The model under review builds one solid part; all positions refer to its coordinate system, in mm. A direction names the side the tool comes from. Give positions to 0.01 mm unless a question says otherwise; leave off trailing zeros. Order: outer loops, then holes, each group sorted by start corner. A loop starts at its lowest first (then second) coordinate and runs counter-clockwise, first axis right, second up. Notation, with made-up numbers: (-15, 69.25) - (10, 69.25) arc R32 cw to (10, 96.25) - close; hole circle Ø4 at (63, 7). An arc over 180 degrees is marked (long way). Use a Markdown table: item, result. Add a question column.
```python
from build123d import *

# Parameters (mm, degrees)
EXTRUDE_1_DEPTH     = 245
CUT_EXTRUDE_1_REACH = 247.917
SKETCH_2_R          = 2
CUT_EXTRUDE_2_REACH = 247.917
SKETCH_3_R          = 6
SKETCH_4_W          = 15
SKETCH_4_H          = 30
CUT_EXTRUDE_3_DEPTH = 2


with BuildPart() as part:
    # 草图1 → 凸台-拉伸1 (new, symmetric)
    with BuildSketch(Plane(origin=(0, 0, 0), x_dir=(1, 0, 0), z_dir=(0, 1, 0))):
        with BuildLine():
            Line((-11, -15), (11, -15))
            ThreePointArc((11, -15), (13.828427125, -13.828427125), (15, -11))
            Line((15, -11), (15, 11))
            ThreePointArc((15, 11), (13.828427125, 13.828427125), (11, 15))
            Line((11, 15), (-11, 15))
            ThreePointArc((-11, 15), (-13.828427125, 13.828427125), (-15, 11))
            Line((-15, 11), (-15, -11))
            ThreePointArc((-15, -11), (-13.828427125, -13.828427125), (-11, -15))
        make_face()
        with BuildLine():
            Line((-11, -13), (11, -13))
            ThreePointArc((11, -13), (12.414213562, -12.414213562), (13, -11))
            Line((13, -11), (13, 11))
            ThreePointArc((13, 11), (12.414213562, 12.414213562), (11, 13))
            Line((11, 13), (-11, 13))
            ThreePointArc((-11, 13), (-12.414213562, 12.414213562), (-13, 11))
            Line((-13, 11), (-13, -11))
            ThreePointArc((-13, -11), (-12.414213562, -12.414213562), (-11, -13))
        make_face(mode=Mode.SUBTRACT)
    extrude(amount=EXTRUDE_1_DEPTH, both=True)

    # 草图2 → 切除-拉伸1 (cut, up to next)
    with BuildSketch(Plane(origin=(0, 0, 0), x_dir=(0, 0, -1), z_dir=(1, 0, 0)), mode=Mode.PRIVATE) as cut_extrude_1_sk1:
        with Locations(Location((0, -100, 0), (0, 0, 180))):
            Circle(SKETCH_2_R)
    cut_extrude_1_tool1 = extrude(cut_extrude_1_sk1.sketch, amount=CUT_EXTRUDE_1_REACH, mode=Mode.PRIVATE) & part.part
    # 草图2 → 切除-拉伸1 (cut, up to next)
    with BuildSketch(Plane(origin=(0, 0, 0), x_dir=(0, 0, -1), z_dir=(1, 0, 0)), mode=Mode.PRIVATE) as cut_extrude_1_sk2:
        with Locations(Location((0, 100, 0), (0, 0, 180))):
            Circle(SKETCH_2_R)
    cut_extrude_1_tool2 = extrude(cut_extrude_1_sk2.sketch, amount=CUT_EXTRUDE_1_REACH, mode=Mode.PRIVATE) & part.part
    add(cut_extrude_1_tool1.solids().sort_by_distance((0, -100, 0))[0], mode=Mode.SUBTRACT)
    add(cut_extrude_1_tool2.solids().sort_by_distance((0, 100, 0))[0], mode=Mode.SUBTRACT)

    # 草图3 → 切除-拉伸2 (cut, up to next)
    with BuildSketch(Plane(origin=(0, 0, 0), x_dir=(0, 0, -1), z_dir=(1, 0, 0)), mode=Mode.PRIVATE) as cut_extrude_2_sk1:
        with Locations((0, -100)):
            Circle(SKETCH_3_R)
    cut_extrude_2_tool1 = extrude(cut_extrude_2_sk1.sketch, amount=-CUT_EXTRUDE_2_REACH, mode=Mode.PRIVATE) & part.part
    # 草图3 → 切除-拉伸2 (cut, up to next)
    with BuildSketch(Plane(origin=(0, 0, 0), x_dir=(0, 0, -1), z_dir=(1, 0, 0)), mode=Mode.PRIVATE) as cut_extrude_2_sk2:
        with Locations((0, 100)):
            Circle(SKETCH_3_R)
    cut_extrude_2_tool2 = extrude(cut_extrude_2_sk2.sketch, amount=-CUT_EXTRUDE_2_REACH, mode=Mode.PRIVATE) & part.part
    add(cut_extrude_2_tool1.solids().sort_by_distance((0, -100, 0))[0], mode=Mode.SUBTRACT)
    add(cut_extrude_2_tool2.solids().sort_by_distance((0, 100, 0))[0], mode=Mode.SUBTRACT)

    # 草图4 → 切除-拉伸3 (cut)
    with BuildSketch(Plane.XY.offset(-15)):
        with Locations((7.5, -100)):
            Rectangle(SKETCH_4_W, SKETCH_4_H)
        with Locations((7.5, 100)):
            Rectangle(SKETCH_4_W, SKETCH_4_H)
    extrude(amount=CUT_EXTRUDE_3_DEPTH, mode=Mode.SUBTRACT)


solid = part.part
```
Q1. Machinability: for faces 1 (the flat face through (0, 3, 13)), 2 (the flat face through (0, 3, -15)), 3 (the cylindrical face through (-13.99, -94.05, 0.78)), which of the approach directions +Z, -Z, +X, -X, +Y, -Y give a long, thin tool a straight path to every point of the face, cutting with its end or side? Answer none if there is none.
Q2. Clearance check with flat-ended pins moving along their axes: P1, Ø3, axis at x = 12.5, y = -98.5, coming from the -Z side; P2, Ø3, axis at y = 100, z = 0, coming from the +X side; P3, Ø1, axis at y = -99.5, z = -14, coming from the +X side; P4, Ø4.5, axis at y = -100, z = 0, coming from the -X side. State where each tip first meets the part, or that it passes through.
Q3. Draft analysis for pull direction X (two halves, no side actions). For faces 4 (the flat face through (-15, 3, 0)), 5 (the flat face through (0, 3, 15)), 6 (the flat face through (15, 3, 0)), 7 (the flat face through (-13, 3, 0)), state which applies: pulls with the +X half, pulls with the -X half, needs draft (parallel to the pull), parting line crosses it, or undercut.
Q4. We need section A-A (x = -5.25). Write out the cut boundary in (y, z), plus the area to 3 significant figures.
Q5. We need section B-B (y = 68). Write out the cut boundary in (x, z), plus the area to 3 significant figures.
Q6. Wall thickness on probe 1 along Y at (x, z) = (-13.9, 0); probe 2 along X at (y, z) = (-109, -1.5): over which ranges is each line inside the solid? List them lowest first.
Here are the results:
| question | item | result |
|---|---|---|
| 1 | face 1 | +Y, -Y |
| 1 | face 2 | -Z, +X, -X, +Y, -Y |
| 1 | face 3 | -X |
| 2 | P1 | z = -13 |
| 2 | P2 | through |
| 2 | P3 | x = 0 |
| 2 | P4 | x = 13 |
| 3 | face 4 | pulls with the -X half |
| 3 | face 5 | needs draft |
| 3 | face 6 | pulls with the +X half |
| 3 | face 7 | undercut |
| 4 | outline | (-245, -15) - (245, -15) - (245, -13) - (-245, -13) - close; (-245, 13) - (245, 13) - (245, 15) - (-245, 15) - close |
| 4 | area | 1,960 mm2 |
| 5 | outline | (-15, -11) arc R4 ccw to (-11, -15) - (11, -15) arc R4 ccw to (15, -11) - (15, 11) arc R4 ccw to (11, 15) - (-11, 15) arc R4 ccw to (-15, 11) - close; hole (-13, -11) arc R2 ccw to (-11, -13) - (11, -13) arc R2 ccw to (13, -11) - (13, 11) arc R2 ccw to (11, 13) - (-11, 13) arc R2 ccw to (-13, 11) - close |
| 5 | area | 214 mm2 |
| 6 | probe 1 | -245 to -106, -94 to 94, 106 to 245 |
| 6 | probe 2 | -15 to -13, 13 to 15 |
